Design review of the part built by this model. Coordinates are the model's own, in mm. Round coordinates to 2 decimals unless told otherwise and drop trailing zeros. Loops run counter-clockwise (first coordinate to the right, second up) from the corner with the lowest first, then second, coordinate; pieces in that order, holes last. Notation, with made-up numbers: M 7.25,26.25 L 48.25,26.25 A13 ccw 48.25,31.25 Z; hole C -7.75,58 d1. An arc over 180 degrees is marked long. Use a Markdown table: item, result.
from build123d import *

# Parameters (mm, degrees)
BOSS_EXTRUDE1_DEPTH = 1.22
SKETCH3_R           = 1.6
CUT_EXTRUDE1_DEPTH  = 246.803551555
SKETCH4_R           = 12
SKETCH4_R_2         = 5
SKETCH4_R_3         = 1.75
SKETCH4_R_4         = 1.6
SKETCH4_R_5         = 6.35
CUT_EXTRUDE2_DEPTH  = 246.803551555


with BuildPart() as part:
    # Sketch1 → Boss-Extrude1 (new body)
    with BuildSketch(Plane(origin=(0, 0, 0), x_dir=(0, 0, -1), z_dir=(1, 0, 0))):
        with BuildLine():
            Line((62.8, 9.646), (-62.8, 9.646))
            ThreePointArc((-62.8, 9.646), (-63.428617928, 9.385617928), (-63.689, 8.757))
            Line((-63.689, 8.757), (-63.689, -236.517))
            ThreePointArc((-63.689, -236.517), (-63.428617928, -237.145617928), (-62.8, -237.406))
            Line((-62.8, -237.406), (62.8, -237.406))
            ThreePointArc((62.8, -237.406), (63.428617928, -237.145617928), (63.689, -236.517))
            Line((63.689, -236.517), (63.689, 8.757))
            ThreePointArc((63.689, 8.757), (63.428617928, 9.385617928), (62.8, 9.646))
        make_face()
    extrude(amount=-BOSS_EXTRUDE1_DEPTH)

    # Sketch3 → Cut-Extrude1 (cut, through all)
    with BuildSketch(Plane(origin=(0, 0, 0), x_dir=(0, 0, -1), z_dir=(1, 0, 0))):
        with Locations((47.5, -107.5)):
            Circle(SKETCH3_R)
        with Locations((-47.5, -107.5)):
            Circle(SKETCH3_R)
        with Locations((47.5, -17.5)):
            Circle(SKETCH3_R)
        with Locations((0, -17.5)):
            Circle(SKETCH3_R)
        with Locations((-47.5, -17.5)):
            Circle(SKETCH3_R)
        with Locations((-47.5, -210.26)):
            Circle(SKETCH3_R)
        with Locations((0, -210.26)):
            Circle(SKETCH3_R)
        with Locations((47.5, -210.26)):
            Circle(SKETCH3_R)
        with Locations((-47.5, -120.26)):
            Circle(SKETCH3_R)
        with Locations((47.5, -120.26)):
            Circle(SKETCH3_R)
    extrude(amount=-CUT_EXTRUDE1_DEPTH, mode=Mode.SUBTRACT)

    # Sketch4 → Cut-Extrude2 (cut, through all)
    with BuildSketch(Plane(origin=(0, 0, 0), x_dir=(0, 0, -1), z_dir=(1, 0, 0))):
        with Locations((25, -48.88)):
            Circle(SKETCH4_R)
        with Locations((-25, -49.13)):
            Circle(SKETCH4_R_2)
        with Locations((35, -183.88)):
            Circle(SKETCH4_R_3)
        with Locations((-5, -183.88)):
            Circle(SKETCH4_R_3)
        with Locations((34.5, -36.88)):
            Circle(SKETCH4_R_4)
        with Locations((15.5, -60.88)):
            Circle(SKETCH4_R_4)
        with Locations((-15, -49.13)):
            Circle(SKETCH4_R_4)
        with Locations((-25, -183.88)):
            Circle(SKETCH4_R_5)
        with BuildLine():
            Line((0.5, -193.88), (29.5, -193.88))
            ThreePointArc((29.5, -193.88), (29.853553391, -193.733553391), (30, -193.38))
            Line((30, -193.38), (30, -174.38))
            ThreePointArc((30, -174.38), (29.853553391, -174.026446609), (29.5, -173.88))
            Line((29.5, -173.88), (0.5, -173.88))
            ThreePointArc((0.5, -173.88), (0.146446609, -174.026446609), (0, -174.38))
            Line((0, -174.38), (0, -193.38))
            ThreePointArc((0, -193.38), (0.146446609, -193.733553391), (0.5, -193.88))
        make_face()
        with BuildLine():
            Line((6.7, -111.800937711), (6.7, -115.959062289))
            ThreePointArc((6.7, -115.959062289), (19.05, -113.88), (6.7, -111.800937711))
        make_face()
        with BuildLine():
            Line((-6.7, -111.800937711), (-6.7, -115.959062289))
            ThreePointArc((-6.7, -115.959062289), (-19.05, -113.88), (-6.7, -111.800937711))
        make_face()
    extrude(amount=-CUT_EXTRUDE2_DEPTH, mode=Mode.SUBTRACT)


solid = part.part
1. Take a section at A-A on z = 25. Give the boundary of the cut face in (x, y), and give its area (3 significant figures).
Check values:
| item | result |
|---|---|
| outline | M -1.22,-237.41 L 0,-237.41 L 0,-190.23 L -1.22,-190.23 Z; M -1.22,-177.53 L 0,-177.53 L 0,-54.13 L -1.22,-54.13 Z; M -1.22,-44.13 L 0,-44.13 L 0,9.65 L -1.22,9.65 Z |
| area | 274 mm² |
2. Take a section at B-B on x = -0.55. Count the separate pieces of the cut face and the enclosed holes in it, and give its area (3 significant figures).
Check values:
| item | result |
|---|---|
| separate pieces | 1 |
| enclosed holes | 21 |
| area | 29,800 mm² |
3. The part is to be moulded in two halves that separate along Y. For faces 1 (the face through (-0.601, -114.13, -19.045)), 2 (the face through (-1.22, -112, 1)), say which applies: pulls with the +Y half, pulls with the -Y half, needs draft (parallel to the pull), parting line crosses it, or undercut.
Check values:
| item | result |
|---|---|
| face 1 | undercut |
| face 2 | needs draft |
4. Wall thickness on line 1 along Z through (x, y) = (-0.7, -120.26); line 2 along Y through (x, z) = (-0.35, 25); line 3 along Y through (x, z) = (-0.9, 47.5): over which ranges is each line inside the solid? List them lowest first. Write a range as from..to.
Check values:
| item | result |
|---|---|
| line 1 | z = -63.69..-49.1, -45.9..45.9, 49.1..63.69 |
| line 2 | y = -237.41..-190.23, -177.53..-54.13, -44.13..9.65 |
| line 3 | y = -237.41..-211.86, -208.66..-121.86, -118.66..-109.1, -105.9..-19.1, -15.9..9.65 |
